from build123d import *

# Parameters (mm, degrees)
F0_W     = 25.4
F0_H     = 25.4
F1_DEPTH = 508
F2_DEPTH = 355.6
F3_W     = 199.9996
F3_H     = 199.9996
F4_DEPTH = 3.175


with BuildPart() as f1:
    # F0 (on Top) → F1 (new body)
    with BuildSketch(Plane.XY):
        with Locations((0.54235, 2.626543)):
            Rectangle(F0_W, F0_H)
    extrude(amount=F1_DEPTH)

    # F0 (on Top) → F2 (join)
    with BuildSketch(Plane.XY):
        with Locations((0.54235, 2.626543)):
            Rectangle(F0_W, F0_H)
    extrude(amount=F2_DEPTH)

    # F3 (on Top) → F4 (join)
    with BuildSketch(Plane.XY):
        with Locations((-93.20364, 47.161473)):
            Rectangle(F3_W, F3_H)
    extrude(amount=F4_DEPTH)


solid = f1.part
Can you work these out from the model? Positions are in its coordinate system, mm. A direction names the side the tool comes from. Give positions to 0.01 mm unless a question says otherwise; leave off trailing zeros. Order: outer loops, then holes, each group sorted by start corner. A loop starts at its lowest first (then second) coordinate and runs counter-clockwise, first axis right, second up. Notation, with made-up numbers: M -21.5,-26 L 8.5,-26 A36 ccw 8.5,13 Z; hole C 32.5,80.25 d3. An arc over 180 degrees is marked long. Use one line per item in the form item = value.
Item 1: If we section it at A-A, the plane y = 9: Write out the boundary of the cut face in (x, z) (3 decimals), and give its area (3 significant figures).
Values follow:
outline = M -193.203,0 L 13.242,0 L 13.242,508 L -12.158,508 L -12.158,3.175 L -193.203,3.175 Z
area = 13,500 mm^2
Item 2: Will these pins go through, and if not, where does the flat tip stop? pin 1 Ø2.5 at (y, z) = (-36, 1.5) entering from +X; pin 2 Ø7.5 at (x, z) = (0.5, 363.5) entering from -Y; pin 3 Ø1.5 at (x, z) = (-9, 325.5) entering from +Y.
Values follow:
pin_1 = 6.8
pin_2 = -10.07
pin_3 = 15.33
Item 3: If we section it at B-B, the plane x = -24.5: Write out the boundary of the cut face in (y, z) (3 decimals), and give its area (3 significant figures).
Values follow:
outline = M -52.838,0 L 147.161,0 L 147.161,3.175 L -52.838,3.175 Z
area = 635 mm^2
Item 4: If we section it at C-C, the plane z = 307: Write out the boundary of the cut face in (x, y).
Values follow:
outline = M -12.16,-10.07 L 13.24,-10.07 L 13.24,15.33 L -12.16,15.33 Z
Item 5: If I drill on line 1 along Z through (x, y) = (-9.5, 92) (3 decimals), over which ranges is the centre line in solid material (lowest first)? Write a range as [from, to].
Values follow:
line_1 = [0, 3.175]
Item 6: For faces 1 (the flat face through (13.242, 2, 250)), 2 (the flat face through (-12.158, 2, 252)), which set-ups out of +Z, -Z, +X, -X, +Y, -Y let a thin tool reach every point of the face, with its end or its side?
Values follow:
face_1 = +Z, -Z, +X, +Y, -Y
face_2 = +Z, -X, +Y, -Y
